```python
from build123d import *

# Parameters (mm, degrees)
PAD_DEPTH       = 25
POCKET_DEPTH    = 12
SKETCH002_R     = 1.5
PAD001_DEPTH    = 6
POCKET001_DEPTH = 2.001
SKETCH004_W     = 2.3
SKETCH004_H     = 10
POCKET002_DEPTH = 9.001
SKETCH005_R     = 1.5
HOLE_DEPTH      = 2.701


with BuildPart() as part:
    # Sketch → Pad (new body)
    with BuildSketch(Plane.XZ):
        Polygon((0, 0), (0, 2), (14, 8), (14, 5), (23, 2), (23, 0), align=None)
    extrude(amount=PAD_DEPTH)

    # Sketch001 (on Face8 of Pad) → Pocket (cut)
    with BuildSketch(Plane.XZ.offset(25)):
        Polygon((0, 2), (14, 2), (14, 8), align=None)
    extrude(amount=-POCKET_DEPTH, mode=Mode.SUBTRACT)

    # Sketch002 (on Face3 of Pocket) → Pad001 (join)
    with BuildSketch(Plane(origin=(-0.724138, 0, 1.689655), x_dir=(-0.919145, 0, -0.393919), z_dir=(-0.393919, 0, 0.919145))):
        with Locations((-8.019385, 8)):
            Circle(SKETCH002_R)
    extrude(amount=PAD001_DEPTH)

    # Sketch003 (on Face4 of Pad001) → Pocket001 (cut, through all)
    with BuildSketch(Plane(origin=(0, 0, 2), x_dir=(-1, 0, 0), z_dir=(0, 0, 1))):
        with BuildLine():
            ThreePointArc((-2.500319, 21.030919), (-4.030919, 22.499681), (-5.499681, 20.969081))
            Line((-5.499681, 14.969081), (-5.499681, 20.969081))
            ThreePointArc((-5.499681, 14.969081), (-3.969081, 13.500319), (-2.500319, 15.030919))
            Line((-2.500319, 15.030919), (-2.500319, 21.030919))
        make_face()
    extrude(amount=-POCKET001_DEPTH, mode=Mode.SUBTRACT)

    # Sketch004 (on Face15 of Pocket001) → Pocket002 (cut, through all)
    with BuildSketch(Plane(origin=(14, 0, 0), x_dir=(0, 0, -1), z_dir=(-1, 0, 0))):
        with Locations((-3.85, 20)):
            Rectangle(SKETCH004_W, SKETCH004_H)
    extrude(amount=-POCKET002_DEPTH, mode=Mode.SUBTRACT)

    # Sketch005 (on Face17 of Pocket002) → Hole (cut, through all)
    with BuildSketch(Plane(origin=(0, 0, 2.7), x_dir=(-1, 0, 0), z_dir=(0, 0, 1))):
        with Locations((-19, 18)):
            Circle(SKETCH005_R)
    extrude(amount=-HOLE_DEPTH, mode=Mode.SUBTRACT)


solid = part.part
```
Build history of the part. All positions in model axes, mm. A direction names the side the tool comes from. Round coordinates to 2 decimals unless told otherwise and drop trailing zeros. Order: outer loops, then holes, each group sorted by start corner. A loop starts at its lowest first (then second) coordinate and runs counter-clockwise, first axis right, second up. Notation, with made-up numbers: (-19, 80) - (16, 80) arc R7 ccw to (16, 84) - close; hole circle Ø4 at (1.5, -15.75). An arc over 180 degrees is marked (long way). Use a Markdown table: item, result.
1) Flat gauge pins, fed straight in: pin 1 Ø4 at (x, y) = (12.5, -4.5) entering from +Z; pin 2 Ø4 at (x, z) = (2.5, 8) entering from +Y; pin 3 Ø9.5 at (x, y) = (5, -21) entering from +Z; pin 4 Ø2.5 at (y, z) = (-20.5, 4) entering from -X. Where does each tip first touch, or does it go through?
Recorded:
| item | result |
|---|---|
| pin 1 | stops at z = 8 |
| pin 2 | stops at y = -6.61 |
| pin 3 | stops at z = 2 |
| pin 4 | passes through |
2) Saw through at B-B on x = 19. Write the cut outline in (y, z).
Recorded:
| item | result |
|---|---|
| outline | (-25, 0) - (-19.5, 0) - (-19.5, 2.7) - (-25, 2.7) - close; (-16.5, 0) - (0, 0) - (0, 3.33) - (-15, 3.33) - (-15, 2.7) - (-16.5, 2.7) - close |
3) Saw through at D-D on x = 8.5. Write the cut outline in (y, z).
Recorded:
| item | result |
|---|---|
| outline | (-25, 0) - (0, 0) - (0, 5.64) - (-13, 5.64) - (-13, 2) - (-25, 2) - close |
4) Saw through at C-C on y = -4.5. Write the cut outline in (x, z), and give its area (4 significant figures).
Recorded:
| item | result |
|---|---|
| outline | (0, 0) - (23, 0) - (23, 2) - (14, 5) - (14, 8) - (0, 2) - close |
| area | 101.5 mm² |
5) Saw through at A-A on y = -18. Write the cut outline in (x, z), and give its area (3 significant figures).
Recorded:
| item | result |
|---|---|
| outline | (0, 0) - (2.5, 0) - (2.5, 2) - (0, 2) - close; (5.5, 0) - (17.5, 0) - (17.5, 2.7) - (14, 2.7) - (14, 2) - (5.5, 2) - close; (20.5, 0) - (23, 0) - (23, 2) - (20.9, 2.7) - (20.5, 2.7) - close |
| area | 37.5 mm² |
6) Tool access for faces 4 (the face through (17, -20, 2.7)), 5 (the face through (10, -13, 4)), 6 (the face through (0, -12, 1)), 7 (the face through (14, -6, 7)), 8 (the face through (5.5, -18, 1)): list every direction of +Z, -Z, +X, -X, +Y, -Y with a clear straight run to the whole face (end or side of a thin tool).
Recorded:
| item | result |
|---|---|
| face 4 | +Z, +X, -X, -Y |
| face 5 | +Z, -X, -Y |
| face 6 | +Z, -Z, -X, +Y, -Y |
| face 7 | +Z, +X, +Y, -Y |
| face 8 | +Z, -Z |
7) Pull direction Y, two halves, no side cores. Call faces 1 (the face through (2.5, -18, 1)), 2 (the face through (12, 0, 2)), 3 (the face through (12, -25, 1)): pulls with the +Y half, pulls with the -Y half, needs draft (parallel to the pull), parting line crosses it, or undercut.
Recorded:
| item | result |
|---|---|
| face 1 | undercut |
| face 2 | pulls with the +Y half |
| face 3 | pulls with the -Y half |
8) Wall check: L1, parallel to X at y = -18, z = 1.2; L2, parallel to X at y = -21, z = 1; L3, parallel to Y at x = 19, z = 1.4. Give the ranges that are in metal, low to high.
Recorded:
| item | result |
|---|---|
| L1 | x = 0 to 2.5, 5.5 to 17.5, 20.5 to 23 |
| L2 | x = 0 to 2.5, 5.5 to 23 |
| L3 | y = -25 to -19.5, -16.5 to 0 |
